Read the model definition and answer for the solid it produces. Units are mm, in the model's axes. A direction names the side the tool comes from. Coordinates: 2 decimals unless noted, no trailing zeros. Write each loop counter-clockwise with the first axis right and the second up, starting at its lowest first coordinate (ties: lowest second). Pieces come first, ordered by that corner, then holes. Notation, with made-up numbers: (67, -21.5) -> (94, -21.5) arc R12 cw to (94, -14.5) -> close; hole circle Ø2 at (-2.75, 63.5). An arc over 180 degrees is marked (long way). Write item = value, one per line. Start each with the question number.
1) Find the intervals of material crossed by line 1 along Z through (x, y) = (6.25, 2); line 2 along Z through (x, y) = (3.5, 6.5); line 3 along Y through (x, z) = (2.5, -0.25), in increasing order. Write a range as from..to.
2) Section C-C (y = 2.75) is taken. Determine the outline of the cut face in (x, z), plus the area to 3 significant figures.
3) A tool of negligible diameter and unlimited length cuts with its end or side. For faces 1 (the face through (6.4, 4.74, -0.4)), 2 (the face through (7, 5.425, 7)), 3 (the face through (6.35, 8.27, -0.44)), from which of +Z, -Z, +X, -X, +Y, -Y can it reach the whole face along a straight path? Write none if from no direction.
4) For a pull along X with two mould halves and no side action, classify faces 4 (the face through (5.395, 7, 7)), 5 (the face through (3.5, 6.901, -0.4)), 6 (the face through (0, 6, 2)) as released by +X, released by -X, zero draft, split by the parting line, or undercut.
5) Section A-A (z = 6) is taken. Determine the outline of the cut face in (x, y) (3 decimals).
6) Section D-D (y = 1.25) is taken. Determine the outline of the cut face in (x, z).
7) Section B-B (y = 6.1) is taken. Determine the outline of the cut face in (x, z) (3 decimals).
8) Flat-ended cylindrical pins translate along their axes: pin 1 Ø3 at (x, y) = (6, 5) entering from +Z; pin 2 Ø0.9 at (x, z) = (1, -0.5) entering from +Y; pin 3 Ø1.1 at (x, z) = (7.5, 8) entering from -Y; pin 4 Ø1.5 at (y, z) = (4.5, 8) entering from -X. Find the tip coordinate at first contact, or state that the pin passes through.
Autodesk Inventor part; units mm, degrees
ref_plane "Work Plane1" through (0, 0, 5) normal (0, 0, 1) x (1, 0, 0)
ref_plane "YZ Plane" through (0, 0, 0) normal (1, 0, 0) x (0, 1, 0)
ref_plane "XZ Plane" through (0, 0, 0) normal (0, 1, 0) x (-1, 0, 0)
sketch "Sketch1" plane through (0, 0, 0) normal (0, 0, 1) x (1, 0, 0)
  line L0 (14.6962, 12.74) -> (14.6962, 0) construction
  line L1 (10.61, 12.2) -> (1.53, 12.2)
  arc A0 (1.53, 12.2) -> (0, 10.67) centre (1.53, 10.67) ccw
  line L2 (0, 10.67) -> (0, 1.53)
  arc A1 (0, 1.53) -> (1.53, 0) centre (1.53, 1.53) ccw
  line L3 (1.53, 0) -> (10.61, 0)
  arc A2 (10.61, 0) -> (12.14, 1.53) centre (10.61, 1.53) ccw
  arc A3 (12.14, 10.67) -> (10.61, 12.2) centre (10.61, 10.67) ccw
  line L4 (12.14, 10.67) -> (12.14, 1.53)
  point P0 (0, 0)
  point P1 (0, 0)
  dimension "d10" = 12.74
ref_plane "Work Plane1" through (0, 0, 5) normal (0, 0, 1) x (1, 0, 0)
sketch "Sketch2" plane through (0, 0, 5) normal (0, 0, 1) x (1, 0, 0)
  line L0 (10.88, 12.74) -> (1.8, 12.74)
  line L1 (10.88, 12.74) -> (1.8, 12.74)
  arc A0 (1.8, 12.74) -> (0, 10.94) centre (1.8, 10.94) ccw
  line L2 (0, 10.94) -> (0, 1.8)
  arc A1 (0, 1.8) -> (1.8, 0) centre (1.8, 1.8) ccw
  line L3 (1.8, 0) -> (10.88, 0)
  arc A2 (10.88, 0) -> (12.68, 1.8) centre (10.88, 1.8) ccw
  line L4 (12.68, 1.8) -> (12.68, 10.94)
  arc A3 (12.68, 10.94) -> (10.88, 12.74) centre (10.88, 10.94) ccw
  circle A4 centre (6.34, 6.37) radius 2.8
  line L5 (5.665, 8.395) -> (7.015, 8.395)
  line L6 (7.015, 4.345) -> (5.665, 4.345)
  line L7 (5.665, 4.345) -> (7.015, 8.395) construction
  line L8 (5.665, 8.395) -> (7.015, 4.345) construction
  line L9 (8.365, 5.695) -> (8.365, 7.045)
  line L10 (4.315, 7.045) -> (4.315, 5.695)
  line L11 (4.315, 5.695) -> (8.365, 7.045) construction
  line L12 (8.365, 5.695) -> (4.315, 7.045) construction
  line L13 (4.315, 5.695) -> (5.665, 5.695)
  line L14 (7.015, 5.695) -> (8.365, 5.695)
  line L15 (5.665, 4.345) -> (5.665, 5.695)
  line L16 (5.665, 7.045) -> (5.665, 8.395)
  line L17 (8.365, 7.045) -> (7.015, 7.045)
  line L18 (5.665, 7.045) -> (4.315, 7.045)
  line L19 (7.015, 8.395) -> (7.015, 7.045)
  line L20 (7.015, 5.695) -> (7.015, 4.345)
  point P0 (0, 0)
  dimension "d3" = 5.6
  dimension "d4" = 4.05
  dimension "d5" = 1.35
  dimension "d6" = 4.05
  dimension "d7" = 1.35
extrude "Extrusion3" add sketch "Sketch1" along normal blind 5
sketch "Sketch3" plane through (0, 0, 5) normal (0, 0, 1) x (1, 0, 0)
  line L0 (10.61, 12.47) -> (1.53, 12.47)
  line L1 (10.61, 12.47) -> (1.53, 12.47)
  arc A0 (1.53, 12.47) -> (-0.27, 10.67) centre (1.53, 10.67) ccw
  line L2 (-0.27, 10.67) -> (-0.27, 1.53)
  arc A1 (-0.27, 1.53) -> (1.53, -0.27) centre (1.53, 1.53) ccw
  line L3 (1.53, -0.27) -> (10.61, -0.27)
  arc A2 (10.61, -0.27) -> (12.41, 1.53) centre (10.61, 1.53) ccw
  line L4 (12.41, 1.53) -> (12.41, 10.67)
  arc A3 (12.41, 10.67) -> (10.61, 12.47) centre (10.61, 10.67) ccw
  circle A4 centre (6.07, 6.1) radius 2.8
  line L5 (5.395, 8.125) -> (6.745, 8.125)
  line L6 (6.745, 4.075) -> (5.395, 4.075)
  line L7 (5.395, 4.075) -> (6.745, 8.125) construction
  line L8 (5.395, 8.125) -> (6.745, 4.075) construction
  line L9 (8.095, 5.425) -> (8.095, 6.775)
  line L10 (4.045, 6.775) -> (4.045, 5.425)
  line L11 (4.045, 5.425) -> (8.095, 6.775) construction
  line L12 (8.095, 5.425) -> (4.045, 6.775) construction
  line L13 (4.045, 5.425) -> (5.395, 5.425)
  line L14 (6.745, 5.425) -> (8.095, 5.425)
  line L15 (5.395, 4.075) -> (5.395, 5.425)
  line L16 (5.395, 6.775) -> (5.395, 8.125)
  line L17 (8.095, 6.775) -> (6.745, 6.775)
  line L18 (5.395, 6.775) -> (4.045, 6.775)
  line L19 (6.745, 8.125) -> (6.745, 6.775)
  line L20 (6.745, 5.425) -> (6.745, 4.075)
  line L21 (10.61, 12.2) -> (1.53, 12.2)
  line L22 (0, 10.67) -> (0, 1.53)
  point P0 (0, 0)
  point P1 (-0.27, -0.27)
  point P2 (6.07, 12.2)
  point P3 (0, 6.1)
  point P4 (6.07, 6.1)
  dimension "d14" = 5.6
  dimension "d15" = 4.05
  dimension "d16" = 1.35
  dimension "d17" = 4.05
  dimension "d18" = 1.35
extrude "Extrusion4" add sketch "Sketch3" along normal blind 4.8 contours A4
sketch "Sketch4" plane through (0, 0, 0) normal (0, 0, -1) x (-1, 0, 0)
  line L0 (-13.9436, 0) -> (-13.9436, 2.266)
  line L1 (-15.5559, 0) -> (-15.5559, 6.84)
  line L2 (-1.53, 0) -> (-10.61, 0)
  line L3 (-11.7556, 9.6007) -> (-0.3844, 9.6007) construction
  line L4 (-0.3844, 9.6007) -> (-0.3844, 6.84) construction
  line L5 (-0.3844, 6.84) -> (-11.7556, 6.84) construction
  line L6 (-11.7556, 6.84) -> (-11.7556, 9.6007) construction
  line L7 (-7.4059, 5.316) -> (-4.7341, 5.316) construction
  line L8 (-4.7341, 5.316) -> (-4.7341, 2.266) construction
  line L9 (-4.7341, 2.266) -> (-7.4059, 2.266) construction
  line L10 (-7.4059, 2.266) -> (-7.4059, 5.316) construction
  line L11 (-8.7186, 6.9007) -> (-9.3925, 6.9007)
  line L12 (-9.3925, 6.9007) -> (-9.3925, 8.6905)
  line L13 (-9.3925, 8.6905) -> (-9.8826, 7.5352)
  line L14 (-9.8826, 7.5352) -> (-10.3465, 7.5352)
  line L15 (-10.3465, 7.5352) -> (-10.8366, 8.6905)
  line L16 (-10.8366, 8.6905) -> (-10.8366, 6.9007)
  line L17 (-10.8366, 6.9007) -> (-11.4755, 6.9007)
  line L18 (-11.4755, 6.9007) -> (-11.4755, 9.6007)
  line L19 (-11.4755, 9.6007) -> (-10.6944, 9.6007)
  line L20 (-10.6944, 9.6007) -> (-10.0949, 8.2682)
  line L21 (-10.0949, 8.2682) -> (-9.4997, 9.6007)
  line L22 (-9.4997, 9.6007) -> (-8.7186, 9.6007)
  line L23 (-8.7186, 9.6007) -> (-8.7186, 6.9007)
  line L24 (-8.4495, 6.9007) -> (-7.5371, 9.6007)
  line L25 (-7.5371, 9.6007) -> (-6.7976, 9.6007)
  line L26 (-6.7976, 9.6007) -> (-5.8852, 6.9007)
  line L27 (-5.8852, 6.9007) -> (-6.5831, 6.9007)
  line L28 (-6.5831, 6.9007) -> (-6.7516, 7.4521)
  line L29 (-6.7516, 7.4521) -> (-7.6006, 7.4521)
  line L30 (-7.6006, 7.4521) -> (-7.7712, 6.9007)
  line L31 (-7.7712, 6.9007) -> (-8.4495, 6.9007)
  line L32 (-6.9004, 7.9422) -> (-7.1761, 8.8349)
  line L33 (-7.1761, 8.8349) -> (-7.454, 7.9422)
  line L34 (-7.454, 7.9422) -> (-6.9004, 7.9422)
  line L35 (-3.1217, 6.9007) -> (-3.9466, 6.9007)
  line L36 (-3.9466, 6.9007) -> (-4.6971, 7.8919)
  line L37 (-4.6971, 7.8919) -> (-4.9421, 7.8919)
  line L38 (-4.9421, 7.8919) -> (-4.9421, 6.9007)
  line L39 (-4.9421, 6.9007) -> (-5.616, 6.9007)
  line L40 (-5.616, 6.9007) -> (-5.616, 9.6007)
  line L41 (-5.616, 9.6007) -> (-4.5308, 9.6007)
  spline S0 degree 2 poles (-4.5308, 9.6007) (-4.3054, 9.6007) (-3.9728, 9.5438) (-3.8306, 9.4563) knots 0 0 0 1 2 2 2
  spline S1 degree 2 poles (-3.8306, 9.4563) (-3.6862, 9.3644) (-3.5155, 9.0778) (-3.5155, 8.859) knots 0 0 0 1 2 2 2
  spline S2 degree 2 poles (-3.5155, 8.859) (-3.5155, 8.5505) (-3.7956, 8.1632) (-4.0297, 8.0494) knots 0 0 0 1 2 2 2
  line L42 (-4.0297, 8.0494) -> (-3.1217, 6.9007)
  spline S3 degree 2 poles (-4.2113, 8.7736) (-4.2113, 8.8765) (-4.2901, 9.0231) (-4.3798, 9.0625) knots 0 0 0 1 2 2 2
  spline S4 degree 2 poles (-4.3798, 9.0625) (-4.4433, 9.0887) (-4.5986, 9.104) (-4.7146, 9.104) knots 0 0 0 1 2 2 2
  line L43 (-4.7146, 9.104) -> (-4.9421, 9.104)
  line L44 (-4.9421, 9.104) -> (-4.9421, 8.3776)
  line L45 (-4.9421, 8.3776) -> (-4.7474, 8.3776)
  spline S5 degree 2 poles (-4.7474, 8.3776) (-4.6074, 8.3776) (-4.4082, 8.4126) (-4.3404, 8.4673) knots 0 0 0 1 2 2 2
  spline S6 degree 2 poles (-4.3404, 8.4673) (-4.2748, 8.5198) (-4.2113, 8.6599) (-4.2113, 8.7736) knots 0 0 0 1 2 2 2
  line L46 (-0.5552, 6.9007) -> (-1.3757, 6.9007)
  line L47 (-1.3757, 6.9007) -> (-2.1087, 7.9969)
  line L48 (-2.1087, 7.9969) -> (-2.2421, 7.8131)
  line L49 (-2.2421, 7.8131) -> (-2.2421, 6.9007)
  line L50 (-2.2421, 6.9007) -> (-2.9204, 6.9007)
  line L51 (-2.9204, 6.9007) -> (-2.9204, 9.6007)
  line L52 (-2.9204, 9.6007) -> (-2.2421, 9.6007)
  line L53 (-2.2421, 9.6007) -> (-2.2421, 8.3951)
  line L54 (-2.2421, 8.3951) -> (-1.3757, 9.6007)
  line L55 (-1.3757, 9.6007) -> (-0.5946, 9.6007)
  line L56 (-0.5946, 9.6007) -> (-1.5573, 8.347)
  line L57 (-1.5573, 8.347) -> (-0.5552, 6.9007)
  line L58 (-4.9219, 4.7104) -> (-6.2245, 2.266)
  line L59 (-6.2245, 2.266) -> (-7.0747, 2.266)
  line L60 (-7.0747, 2.266) -> (-5.7128, 4.7401)
  line L61 (-5.7128, 4.7401) -> (-7.1662, 4.7401)
  line L62 (-7.1662, 4.7401) -> (-7.1662, 5.316)
  line L63 (-7.1662, 5.316) -> (-4.9219, 5.316)
  line L64 (-4.9219, 5.316) -> (-4.9219, 4.7104)
  point P0 (0, 0)
  point P1 (-6.07, 0)
  point P2 (-6.07, 2.266)
  point P3 (-6.07, 6.84)
  point P4 (-6.07, 2.266)
  dimension "d21" = 2.266
  dimension "d22" = 6.84
extrude "Extrusion5" add sketch "Sketch4" along normal blind 0.9
properties part number "IPC MARK 7 key"
Answer key:
q1.line_1 = 0..5
q1.line_2 = 0..9.8
q1.line_3 = 6.9..9.6
q2.outline = (0, 0) -> (5.97, 0) -> (5.97, -0.9) -> (6.81, -0.9) -> (6.81, 0) -> (12.14, 0) -> (12.14, 5) -> (0, 5) -> close
q2.area = 61.5 mm^2
q3.face_1 = -Z, +X
q3.face_2 = +Z
q3.face_3 = -Z, +Y
q4.face_4 = undercut
q4.face_5 = zero draft
q4.face_6 = released by -X
q5.outline = circle Ø5.6 at (6.07, 6.1); hole (4.045, 5.425) -> (5.395, 5.425) -> (5.395, 4.075) -> (6.745, 4.075) -> (6.745, 5.425) -> (8.095, 5.425) -> (8.095, 6.775) -> (6.745, 6.775) -> (6.745, 8.125) -> (5.395, 8.125) -> (5.395, 6.775) -> (4.045, 6.775) -> close
q6.outline = (0.03, 0) -> (12.11, 0) -> (12.11, 5) -> (0.03, 5) -> close
q7.outline = (0, 0) -> (12.14, 0) -> (12.14, 5) -> (8.87, 5) -> (8.87, 9.8) -> (8.095, 9.8) -> (8.095, 5) -> (4.045, 5) -> (4.045, 9.8) -> (3.27, 9.8) -> (3.27, 5) -> (0, 5) -> close
q8.pin_1 = 9.8
q8.pin_2 = 9.6
q8.pin_3 = 3.44
q8.pin_4 = 3.4
